Check sheet for the drawn part. Datum: minimum x, y, z corner. Units: mm. Give positions to 0.01 mm unless a question says otherwise; leave off trailing zeros. Use a Markdown table: item, result. Add a question column.
1. Depth check by flat-ended pin: P1, Ø1.9, axis at y = 3, z = 52, coming from the +X side. Enter the tip coordinate at first touch or a pass-through.
2. Cross-section at C-C on y = 2. Count the separate pieces of the cut face and the enclosed holes in it, and give its area (3 significant figures).
3. Draft check along Y on the marked faces 1 and 2. Enter one of: pulls with the +Y half, pulls with the -Y half, needs draft (parallel to the pull), parting line crosses it, or undercut.
4. Material ranges on L1, parallel to X at y = 1.5, z = 95.25 (1 decimal); L2, parallel to Z at x = 22, y = 0.75; L3, parallel to Z at x = 65, y = 5, recorded low to high.
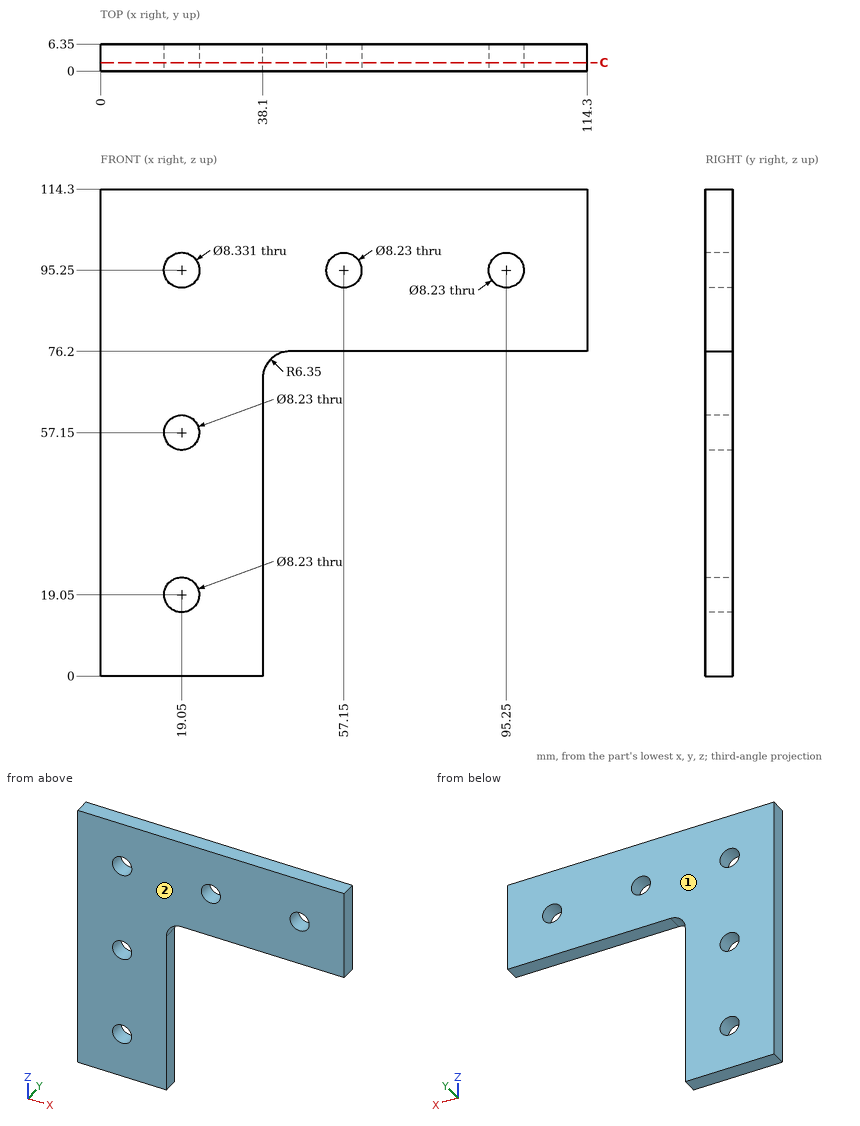
Values found:
| question | item | result |
|---|---|---|
| 1 | P1 | stops at x = 38.1 |
| 2 | separate pieces | 1 |
| 2 | enclosed holes | 5 |
| 2 | area | 7,000 mm2 |
| 3 | face 1 | pulls with the +Y half |
| 3 | face 2 | pulls with the -Y half |
| 4 | L1 | x = 0 to 14.9, 23.2 to 53, 61.3 to 91.1, 99.4 to 114.3 |
| 4 | L2 | z = 0 to 16.18, 21.92 to 54.28, 60.02 to 92.31, 98.19 to 114.3 |
| 4 | L3 | z = 76.2 to 114.3 |
